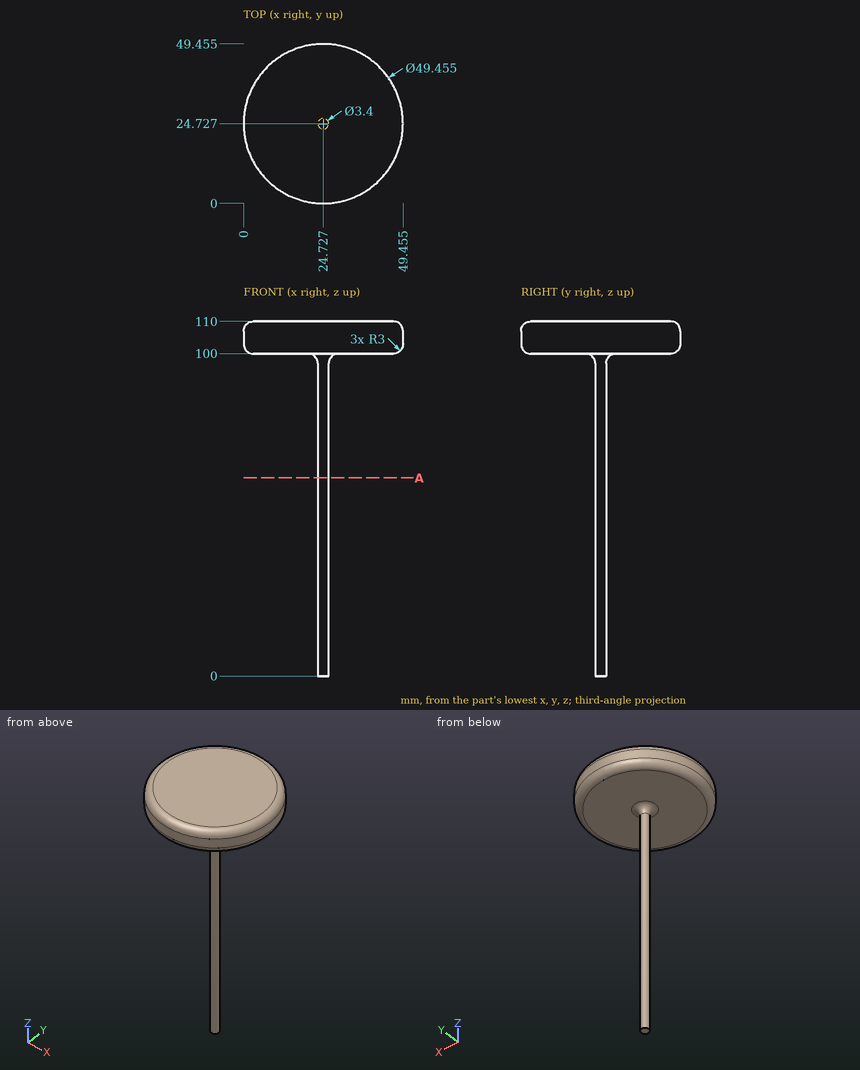
Print and shaded views of the part. All mm, measured from the part's lowest x, y and z. Give positions to 0.01 mm unless a question says otherwise; leave off trailing zeros. Loops run counter-clockwise (first coordinate to the right, second up) from the corner with the lowest first, then second, coordinate; pieces in that order, holes last. Notation, with made-up numbers: (72, -20.5) -> (80, -20.5) arc R19 ccw to (80, -7.5) -> close; hole circle Ø11 at (-2, 63.5). An arc over 180 degrees is marked (long way). Answer in a Markdown table with one row per item.
Item 1: Probe line 1 along Z through (x, y) = (24, 31); line 2 along Y through (x, z) = (25, 105); line 3 along Y through (x, z) = (24, 100.5) (1 decimal). List the from-to ranges inside material, lowest first. Write a range as [from, to].
Findings below:
| item | result |
|---|---|
| line 1 | z = [100, 110] |
| line 2 | y = [0, 49.45] |
| line 3 | y = [1.4, 48.1] |
Item 2: Flat gauge pins, fed straight in: P1, Ø6, axis at x = 29, z = 56, coming from the +Y side (1 decimal); P2, Ø10, axis at x = 22, y = 39, coming from the -Z side; P3, Ø12, axis at y = 18.5, z = 88, coming from the -X side; P4, Ø13, axis at x = 24.5, y = 32, coming from the -Z side. Where does each tip first touch, or does it go through?
Findings below:
| item | result |
|---|---|
| P1 | stops at y = 25.9 |
| P2 | stops at z = 100 |
| P3 | stops at x = 23.04 |
| P4 | stops at z = 0 |
Item 3: Slice it at A-A on z = 61.5. Write the cut outline in (x, y).
Findings below:
| item | result |
|---|---|
| outline | circle Ø3.4 at (24.73, 24.73) |
